```python
from build123d import *

# Parameters (mm, degrees)
EXTRUDE_1_DEPTH     = 2.5
SKETCH_2_R          = 0.5
CUT_EXTRUDE_1_DEPTH = 8
SKETCH_3_R          = 0.6
EXTRUDE_2_DEPTH     = 8
FILLET_1_R          = 0.5


with BuildPart() as part:
    # 草图1 → 凸台-拉伸1 (new body)
    with BuildSketch(Plane.XY):
        Polygon((1.315447425, 1.536749297), (11.975701463, -4.617951242), (10.725701463, -6.783014751), (2.065447425, -1.783014751), (-7.934552575, -1.783014751), (-7.934552575, 1.536749297), align=None)
    extrude(amount=EXTRUDE_1_DEPTH)

    # 草图2 → 切除-拉伸1 (cut)
    with BuildSketch(Plane(origin=(10.981407641, -6.340118658, 0), x_dir=(0, 0, -1), z_dir=(0.8660254037844386, -0.5, 0))):
        with Locations(Location((-1.25, 0.738587643, 0), (0, 0, 90))):
            Circle(SKETCH_2_R)
    extrude(amount=-CUT_EXTRUDE_1_DEPTH, mode=Mode.SUBTRACT)

    # 草图3 → 凸台-拉伸2 (add)
    with BuildSketch(Plane.ZY.offset(7.934552575)):
        with Locations((1.25, -0.123132727)):
            Circle(SKETCH_3_R)
    extrude(amount=EXTRUDE_2_DEPTH)

    # 圆角1
    fillet_1_edges = [part.edges().sort_by_distance(p)[0] for p in [
        (2.065447425, -1.783014751, 1.25),
        (-7.934552575, -1.783014751, 1.25),
        (-7.934552575, 1.536749297, 1.25),
        (1.315447425, 1.536749297, 1.25),
        (11.975701463, -4.617951242, 1.25),
        (10.725701463, -6.783014751, 1.25),
        (6.645574444, -1.540600973, 2.5),
        (-3.309552575, 1.536749297, 2.5),
        (-7.934552575, -0.123132727, 2.5),
        (-2.934552575, -1.783014751, 2.5),
        (6.395574444, -4.283014751, 2.5),
        (-2.934552575, -1.783014751, 0),
        (-7.934552575, -0.123132727, 0),
        (-3.309552575, 1.536749297, 0),
        (6.645574444, -1.540600973, 0),
        (11.350701463, -5.700482996, 0),
        (6.395574444, -4.283014751, 0),
        (11.350701463, -5.700482996, 2.5),
    ]]
    fillet(fillet_1_edges, radius=FILLET_1_R)


solid = part.part
```
Geometry check sheet. Reference: the model listing, model coordinates, mm. A direction names the side the tool comes from. Coordinates: 2 decimals unless noted, no trailing zeros. Order: outer loops, then holes, each group sorted by start corner. A loop starts at its lowest first (then second) coordinate and runs counter-clockwise, first axis right, second up. Notation, with made-up numbers: (-14.5, 72.25) - (37.5, 72.25) arc R11 cw to (37.5, 77.25) - close; hole circle Ø2 at (40.5, 12.5). An arc over 180 degrees is marked (long way). Answer as a JSON object with one key per item and string values. Group by question number.
Item 1: Sectioned sample at C-C, the plane x = -9.75. Record the cut outline in (y, z).
Item 2: Draft check along Y on faces 4 (the face through (-11.88, 0.06, 1.82)), 5 (the face through (6.487, -1.613, 0.15)), 6 (the face through (4.419, -1.707, 1.257)). Enter one of: +Y half, -Y half, draft (parallel to the pull), parting line (faces both ways), or undercut.
Item 3: Sectioned sample at A-A, the plane x = -0.75. Record the cut outline in (y, z), and give its area (3 significant figures).
Item 4: Scan lines: probe 1 along Y at (x, z) = (-1.5, 0.6); probe 2 along Z at (x, y) = (9, -4.5); probe 3 along Y at (x, z) = (7.5, 1.5). Record each from-to range of solid material in increasing order.
Item 5: Tool access check on faces 1 (the face through (11.22, -5.64, 0.15)), 2 (the face through (-7.935, -1, 1)), 3 (the face through (-3, -1.783, 1)). Record the directions out of +Z, -Z, +X, -X, +Y, -Y that give a thin tool (end or side, any length) a straight path to the whole face; none if there is none.
Item 6: Sectioned sample at B-B, the plane z = 1.25. Record the cut outline in (x, y).
Item 7: Depth check by flat-ended pin: pin 1 Ø0.5 at (x, z) = (-0.5, 1.5) entering from -Y. Enter the tip coordinate at first touch or a pass-through.
Resolved:
{
 "1": {"outline": "circle Ø1.2 at (-0.12, 1.25)"},
 "2": {"face 4": "parting line", "face 5": "+Y half", "face 6": "undercut"},
 "3": {"outline": "(-1.78, 0.5) arc R0.5 ccw to (-1.28, 0) - (1.04, 0) arc R0.5 ccw to (1.54, 0.5) - (1.54, 2) arc R0.5 ccw to (1.04, 2.5) - (-1.28, 2.5) arc R0.5 ccw to (-1.78, 2) - close", "area": "8.08 mm^2"},
 "4": {"probe 1": "-1.78 to 1.54", "probe 2": "0 to 0.77, 1.73 to 2.5", "probe 3": "-4.92 to -3.98, -2.98 to -2.03"},
 "5": {"face 1": "-Z, +X, -Y", "face 2": "-X", "face 3": "+Z, -Z, -X, -Y"},
 "6": {"outline": "(-15.93, -0.72) - (-7.93, -0.72) - (-7.93, -1.28) arc R0.5 ccw to (-7.43, -1.78) - (1.93, -1.78) arc R0.5 cw to (2.18, -1.85) - (10.29, -6.53) arc R0.5 ccw to (10.98, -6.35) - (11.1, -6.13) - (4.17, -2.13) - (4.67, -1.27) - (11.6, -5.27) - (11.73, -5.05) arc R0.5 ccw to (11.54, -4.37) - (1.43, 1.47) arc R0.5 ccw to (1.18, 1.54) - (-7.43, 1.54) arc R0.5 ccw to (-7.93, 1.04) - (-7.93, 0.48) - (-15.93, 0.48) - close"},
 "7": {"pin 1": "y = -1.78"}
}
